Can you work these out from the model? Positions are in its coordinate system, mm. A direction names the side the tool comes from. Round coordinates to 2 decimals unless told otherwise and drop trailing zeros. Loops run counter-clockwise (first coordinate to the right, second up) from the corner with the lowest first, then second, coordinate; pieces in that order, holes last.
```python
from build123d import *

# Parameters (mm, degrees)
SKETCH1_R           = 2.5
BOSS_EXTRUDE1_DEPTH = 50
FILLET1_R           = 1.47
SKETCH2_R           = 1.5
CUT_EXTRUDE1_DEPTH  = 53.850827808
SKETCH3_R           = 1.5
CUT_EXTRUDE2_DEPTH  = 53.850827903


with BuildPart() as part:
    # Sketch1 → Boss-Extrude1 (new body)
    with BuildSketch(Plane.XY):
        Polygon((2.860553032, 3.9), (6, 7.039446968), (6, 8.2), (3.1, 8.2), (3.1, 10), (10, 10), (10, 3.1), (8.2, 3.1), (8.2, 6), (7.039446968, 6), (3.9, 2.860553032), (3.9, 0), (3.9, -2.860553032), (7.039446968, -6), (8.2, -6), (8.2, -3.1), (10, -3.1), (10, -10), (3.1, -10), (3.1, -8.2), (6, -8.2), (6, -7.039446968), (2.860553032, -3.9), (0, -3.9), (-2.860553032, -3.9), (-6, -7.039446968), (-6, -8.2), (-3.1, -8.2), (-3.1, -10), (-10, -10), (-10, -3.1), (-8.2, -3.1), (-8.2, -6), (-7.039446968, -6), (-3.9, -2.860553032), (-3.9, 0), (-3.9, 2.860553032), (-7.039446968, 6), (-8.2, 6), (-8.2, 3.1), (-10, 3.1), (-10, 10), (-3.1, 10), (-3.1, 8.2), (-6, 8.2), (-6, 7.039446968), (-2.860553032, 3.9), (0, 3.9), align=None)
        Circle(SKETCH1_R, mode=Mode.SUBTRACT)
    extrude(amount=BOSS_EXTRUDE1_DEPTH)

    # Fillet1
    fillet1_edges = [part.edges().sort_by_distance(p)[0] for p in [
        (10, -10, 25),
        (-10, -10, 25),
        (-10, 10, 25),
        (10, 10, 25),
    ]]
    fillet(fillet1_edges, radius=FILLET1_R)

    # Sketch2 → Cut-Extrude1 (cut, through all)
    with BuildSketch(Plane.XZ.offset(3.9)):
        with Locations((0, 40)):
            Circle(SKETCH2_R)
    extrude(amount=-CUT_EXTRUDE1_DEPTH, mode=Mode.SUBTRACT)

    # Sketch3 → Cut-Extrude2 (cut, through all)
    with BuildSketch(Plane(origin=(0, 3.9, 0), x_dir=(1, 0, 0), z_dir=(0, 1, 0))):
        with Locations(Location((0, -10, 0), (0, 0, 180))):
            Circle(SKETCH3_R)
    extrude(amount=-CUT_EXTRUDE2_DEPTH, mode=Mode.SUBTRACT)


solid = part.part
```
(1) Which directions (+Z, -Z, +X, -X, +Y, -Y) give clear straight access to the entire face, cutting with the end or side of a thin tool? Please do faces 5 (the flat face through (3.1, -9, 25)), 6 (the flat face through (6, 8, 25)), 7 (the flat face through (9, -3.1, 25)), 8 (the flat face through (0, 3.9, 25)).
(2) We'd pull the mould along X, two halves only. Please class faces 1 (the flat face through (10, 6, 25)), 2 (the cylindrical face through (-9.56, 9.58, 25.35)), 3 (the flat face through (-8.2, -5, 25)), 4 (the flat face through (-6, -8, 25)): released by +X, released by -X, zero draft, split by the parting line, or undercut.
(3) For pin 1 (5 mm diameter, centred on x = 0, z = 10, fed in from +Y); pin 2 (1 mm diameter, centred on y = -2, z = 34.5, fed in from +X), each with a flat end and sliding along its axis, tell me the tip position at first contact or that it passes through.
(4) Suppose I cut it at A-A (x = 0). Write out the boundary of the cut face in (y, z), then the cut area to 3 significant figures.
(5) Suppose I cut it at B-B (y = 0). Write out the boundary of the cut face in (x, z).
(6) Suppose I cut it at C-C (y = -4.5). Write out the boundary of the cut face in (x, z).
(7) If I drill on line 1 (Z direction, x = 0, y = 3); line 2 (Y direction, x = -3.5, z = 11.5); line 3 (X direction, y = 2.6, z = 10), over which ranges is the centre line in solid material (lowest first)?
Check result:
1. face 5: +Z, -Z, -Y
1. face 6: +Z, -Z
1. face 7: +Z, -Z, +X
1. face 8: +Z, -Z, +Y
2. face 1: released by +X
2. face 2: released by -X
2. face 3: undercut
2. face 4: undercut
3. pin 1: stops at y = 3.9
3. pin 2: stops at x = 3.9
4. outline: (-3.9, 0) - (-2.5, 0) - (-2.5, 8.5) - (-3.9, 8.5) - close; (-3.9, 11.5) - (-2.5, 11.5) - (-2.5, 38.5) - (-3.9, 38.5) - close; (-3.9, 41.5) - (-2.5, 41.5) - (-2.5, 50) - (-3.9, 50) - close; (2.5, 0) - (3.9, 0) - (3.9, 8.5) - (2.5, 8.5) - close; (2.5, 11.5) - (3.9, 11.5) - (3.9, 38.5) - (2.5, 38.5) - close; (2.5, 41.5) - (3.9, 41.5) - (3.9, 50) - (2.5, 50) - close
4. area: 123 mm2
5. outline: (-3.9, 0) - (-2.5, 0) - (-2.5, 50) - (-3.9, 50) - close; (2.5, 0) - (3.9, 0) - (3.9, 50) - (2.5, 50) - close
6. outline: (-10, 0) - (-8.2, 0) - (-8.2, 50) - (-10, 50) - close; (-5.54, 0) - (-3.46, 0) - (-3.46, 50) - (-5.54, 50) - close; (3.46, 0) - (5.54, 0) - (5.54, 50) - (3.46, 50) - close; (8.2, 0) - (10, 0) - (10, 50) - (8.2, 50) - close
7. line 1: z = 0 to 8.5, 11.5 to 38.5, 41.5 to 50
7. line 2: y = -10 to -8.2, -4.54 to 4.54, 8.2 to 10
7. line 3: x = -3.9 to -1.5, 1.5 to 3.9
